Check sheet for the drawn part. Datum: minimum x, y, z corner. Units: mm. A direction names the side the tool comes from. Round coordinates to 2 decimals unless told otherwise and drop trailing zeros. Write each loop counter-clockwise with the first axis right and the second up, starting at its lowest first coordinate (ties: lowest second). Pieces come first, ordered by that corner, then holes. Notation, with made-up numbers: (34.25, 50) - (42.25, 50) arc R10 ccw to (42.25, 64) - close; hole circle Ø3 at (50, -25). An arc over 180 degrees is marked (long way). Write each question's results on one line, items separated by ' | '.
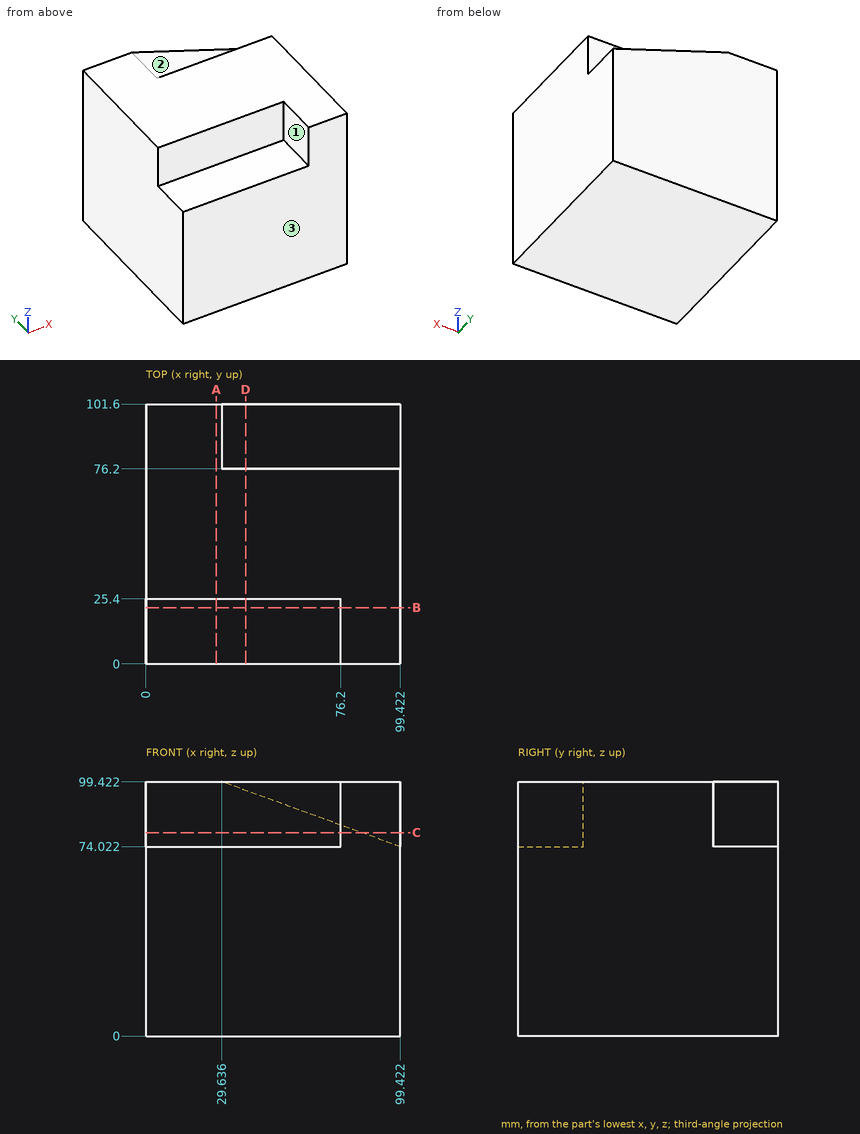
(1) Section check C-C (z = 79.5). Record the cut outline in (x, y).
Answer:
outline: (0, 25.4) - (76.2, 25.4) - (76.2, 0) - (99.42, 0) - (99.42, 76.2) - (84.37, 76.2) - (84.37, 101.6) - (0, 101.6) - close
(2) Section check A-A (x = 27.5). Record the cut outline in (y, z).
Answer:
outline: (0, 0) - (101.6, 0) - (101.6, 99.42) - (25.4, 99.42) - (25.4, 74.02) - (0, 74.02) - close
(3) Section check B-B (y = 22). Record the cut outline in (x, z), plus the area to 3 significant figures.
Answer:
outline: (0, 0) - (99.42, 0) - (99.42, 99.42) - (76.2, 99.42) - (76.2, 74.02) - (0, 74.02) - close | area: 7,950 mm2
(4) Thickness scan on L1, parallel to Y at x = 37.5, z = 81; L2, parallel to Y at x = 89, z = 83.5; L3, parallel to X at y = 25, z = 81. Record the ranges inside material, lowest first.
Answer:
L1: 25.4 to 101.6 | L2: 0 to 76.2 | L3: 76.2 to 99.42
(5) Go/stop test with flat-tipped pins: pin 1 Ø7.5 at (y, z) = (9, 89.5) entering from -X; pin 2 Ø20.5 at (x, y) = (31, 7.5) entering from +Z; pin 3 Ø1.5 at (x, y) = (82, 78.5) entering from +Z. Record where each tip stops, or that it passes through.
Answer:
pin 1: x = 76.2 | pin 2: z = 74.02 | pin 3: z = 80.64
(6) Section check D-D (x = 39). Record the cut outline in (y, z), plus the area to 3 significant figures.
Answer:
outline: (0, 0) - (101.6, 0) - (101.6, 96.01) - (76.2, 96.01) - (76.2, 99.42) - (25.4, 99.42) - (25.4, 74.02) - (0, 74.02) - close | area: 9,370 mm2
(7) Set-up check for the marked faces 1, 2 and 3: record each of +Z, -Z, +X, -X, +Y, -Y from which the full face is reachable in a straight line by a thin tool's end or side.
Answer:
face 1: +Z, -X, -Y | face 2: +Z, +X, +Y | face 3: +Z, -Z, +X, -X, -Y
